from build123d import *

# Parameters (mm, degrees)
SKETCH1_W            = 15.8
SKETCH1_H            = 3.2
BOSS_EXTRUDE1_DEPTH  = 15.8
SKETCH2_R            = 2.4
BOSS_EXTRUDE2_DEPTH  = 1.6
LPATTERN1_COUNT      = 2
LPATTERN1_PITCH      = 8
LPATTERN1_COUNT_DIR2 = 4
LPATTERN1_PITCH_DIR2 = 8
SHELL1_T             = -1.2
SKETCH4_R            = 3.25
SKETCH4_R_2          = 2.4
BOSS_EXTRUDE3_DEPTH  = 1.8
SKETCH6_R            = 2.4
CUT_EXTRUDE1_DEPTH   = 23.519325034
SKETCH11_R           = 1.55
BOSS_EXTRUDE5_DEPTH  = 5
BOSS_EXTRUDE7_REACH  = 28.558
SKETCH14_R           = 1.5


with BuildPart() as part:
    # Sketch1 → Boss-Extrude1 (new body)
    with BuildSketch(Plane.XY):
        with Locations((7.9, 1.6)):
            Rectangle(SKETCH1_W, SKETCH1_H)
    extrude(amount=-BOSS_EXTRUDE1_DEPTH)

    # Sketch2 → Boss-Extrude2 (add)
    with BuildSketch(Plane(origin=(0, 3.2, 0), x_dir=(1, 0, 0), z_dir=(0, 1, 0))):
        with Locations(Location((3.9, 3.9, 0), (0, 0, 270))):
            Circle(SKETCH2_R)
    boss_extrude2 = extrude(amount=BOSS_EXTRUDE2_DEPTH)

    # LPattern1: Boss-Extrude2 2 × 4, 4 skipped
    with Locations(*[(j * LPATTERN1_PITCH_DIR2, 0, -i * LPATTERN1_PITCH) for i in range(LPATTERN1_COUNT) for j in range(LPATTERN1_COUNT_DIR2) if (i, j) not in ((0, 0), (0, 2), (0, 3), (1, 2), (1, 3))]):
        add(boss_extrude2)

    # Shell1
    shell1_openings = [part.faces().sort_by_distance(p)[0] for p in [
        (7.9, 0, -7.9),
    ]]
    offset(amount=SHELL1_T, openings=shell1_openings, kind=Kind.INTERSECTION)

    # Sketch4 → Boss-Extrude3 (add)
    with BuildSketch(Plane.XZ.offset(-2)):
        with Locations(Location((7.9, -7.9, 0), (0, 0, 90))):
            Circle(SKETCH4_R)
        with Locations(Location((7.9, -7.9, 0), (0, 0, 270))):
            Circle(SKETCH4_R_2, mode=Mode.SUBTRACT)
    extrude(amount=BOSS_EXTRUDE3_DEPTH)

    # Sketch6 → Cut-Extrude1 (cut, through all)
    with BuildSketch(Plane.XZ.offset(-2)):
        with Locations(Location((7.9, -7.9, 0), (0, 0, 90))):
            Circle(SKETCH6_R)
    extrude(amount=-CUT_EXTRUDE1_DEPTH, mode=Mode.SUBTRACT)

    # Sketch11 → Boss-Extrude5 (add)
    with BuildSketch(Plane.XY):
        with Locations((8.05, 1.6)):
            Circle(SKETCH11_R)
    extrude(amount=BOSS_EXTRUDE5_DEPTH)


with BuildPart() as body_2:
    # Sketch12 → Revolve1 (revolve)
    with BuildSketch(Plane.XY.offset(7.55)):
        with BuildLine():
            Line((8.05, 4.4), (8.05, -1.2))
            ThreePointArc((8.05, -1.2), (5.25, 1.6), (8.05, 4.4))
        make_face()
    revolve(axis=Axis((8.05, 3.15, 7.55), (0, -1, 0)))

    # Sketch14 → Boss-Extrude7 (add, up to next)
    with BuildSketch(Plane.XY.offset(5), mode=Mode.PRIVATE) as boss_extrude7_sk1:
        with Locations((8.05, 1.6)):
            Circle(SKETCH14_R)
    boss_extrude7_tool1 = extrude(boss_extrude7_sk1.sketch, amount=BOSS_EXTRUDE7_REACH, mode=Mode.PRIVATE) - body_2.part

    add(part.part)  # Boss-Extrude7 merges part
    add(boss_extrude7_tool1.solids().sort_by_distance((8.05, 1.6, 5))[0])


solid = body_2.part
Geometry check sheet. Reference: the model listing, model coordinates, mm. A direction names the side the tool comes from. Give positions to 0.01 mm unless a question says otherwise; leave off trailing zeros. Loops run counter-clockwise (first coordinate to the right, second up) from the corner with the lowest first, then second, coordinate; pieces in that order, holes last. Notation, with made-up numbers: M 76.25,-29.75 L 92.25,-29.75 A16 ccw 92.25,-11.75 Z; hole C 63,47.25 d5. An arc over 180 degrees is marked long. Write each question's results on one line, items separated by ' | '.
1) Tool access check on faces 1 (the face through (12, 3.6, -4)), 2 (the face through (4, 4.8, -4)), 3 (the face through (14.28, 3.99, -12.21)). Record the directions out of +Z, -Z, +X, -X, +Y, -Y that give a thin tool (end or side, any length) a straight path to the whole face; none if there is none.
Answers follow:
face 1: -Y | face 2: +Z, -Z, +X, -X, +Y | face 3: +Y
2) Section check B-B, the plane x = 3.9. Record the boundary of the cut face in (y, z), plus the area to 3 significant figures.
Answers follow:
outline: M 0,-15.8 L 3.2,-15.8 L 3.2,-14.3 L 4.8,-14.3 L 4.8,-9.5 L 3.2,-9.5 L 3.2,-6.3 L 4.8,-6.3 L 4.8,-1.5 L 3.2,-1.5 L 3.2,0 L 0,0 L 0,-1.2 L 2,-1.2 L 2,-2.7 L 3.6,-2.7 L 3.6,-5.1 L 2,-5.1 L 2,-10.7 L 3.6,-10.7 L 3.6,-13.1 L 2,-13.1 L 2,-14.6 L 0,-14.6 Z | area: 31.4 mm2
3) Thickness scan on line 1 (X direction, y = 3.05, z = -3.9); line 2 (Z direction, x = 4, y = 2.75); line 3 (X direction, y = 2.95, z = -7.9). Record the ranges inside material, lowest first.
Answers follow:
line 1: 0 to 2.7, 5.1 to 10.7, 13.1 to 15.8 | line 2: -15.8 to -13.1, -10.7 to -5.1, -2.7 to 0 | line 3: 0 to 5.5, 10.3 to 15.8
4) Section check A-A, the plane z = -8.5. Record the boundary of the cut face in (x, y), plus the area to 3 significant figures.
Answers follow:
outline: M 0,0 L 1.2,0 L 1.2,2 L 4.71,2 L 4.71,0.2 L 5.58,0.2 L 5.58,3.2 L 0,3.2 Z; M 10.22,0.2 L 11.09,0.2 L 11.09,2 L 14.6,2 L 14.6,0 L 15.8,0 L 15.8,3.2 L 10.22,3.2 Z | area: 21.3 mm2
5) Gauge pin test, flat ends, axial feed: pin 1 (3 mm diameter, centred on x = 11.9, z = -11.9, fed in from -Y); pin 2 (7 mm diameter, centred on x = 9.5, z = -8.5, fed in from -Y); pin 3 (1.4 mm diameter, centred on x = 3.9, z = -3.9, fed in from -Y); pin 4 (4.5 mm diameter, centred on x = 11.5, z = -6.5, fed in from +Y). Record the tip position at first contact, or that the pin passes through.
Answers follow:
pin 1: y = 2 | pin 2: y = 0.2 | pin 3: y = 3.6 | pin 4: y = 4.8
6) Section check C-C, the plane x = 7.5. Record the boundary of the cut face in (y, z), plus the area to 3 significant figures.
Answers follow:
outline: M 0,-15.8 L 3.2,-15.8 L 3.2,-10.27 L 0.2,-10.27 L 0.2,-11.13 L 2,-11.13 L 2,-14.6 L 0,-14.6 Z; M 0,-1.2 L 2,-1.2 L 2,-4.67 L 0.2,-4.67 L 0.2,-5.53 L 3.2,-5.53 L 3.2,0 L 3.05,0 L 3.05,5 L 3,5 L 3,5.19 A2.75 ccw long 0.2,5.19 L 0.2,5 L 0.15,5 L 0.15,0 L 0,0 Z | area: 59.1 mm2
7) Release check for a two-part mould opening along Z. For faces 4 (the face through (1.2, 1, -8)), 5 (the face through (1, 0, -8)) record: +Z half, -Z half, draft (parallel to the pull), parting line (faces both ways), or undercut.
Answers follow:
face 4: undercut | face 5: draft
8) Section check D-D, the plane z = -11.9. Record the boundary of the cut face in (x, y).
Answers follow:
outline: M 0,0 L 1.2,0 L 1.2,2 L 2.7,2 L 2.7,3.6 L 5.1,3.6 L 5.1,2 L 10.7,2 L 10.7,3.6 L 13.1,3.6 L 13.1,2 L 14.6,2 L 14.6,0 L 15.8,0 L 15.8,3.2 L 14.3,3.2 L 14.3,4.8 L 9.5,4.8 L 9.5,3.2 L 6.3,3.2 L 6.3,4.8 L 1.5,4.8 L 1.5,3.2 L 0,3.2 Z
